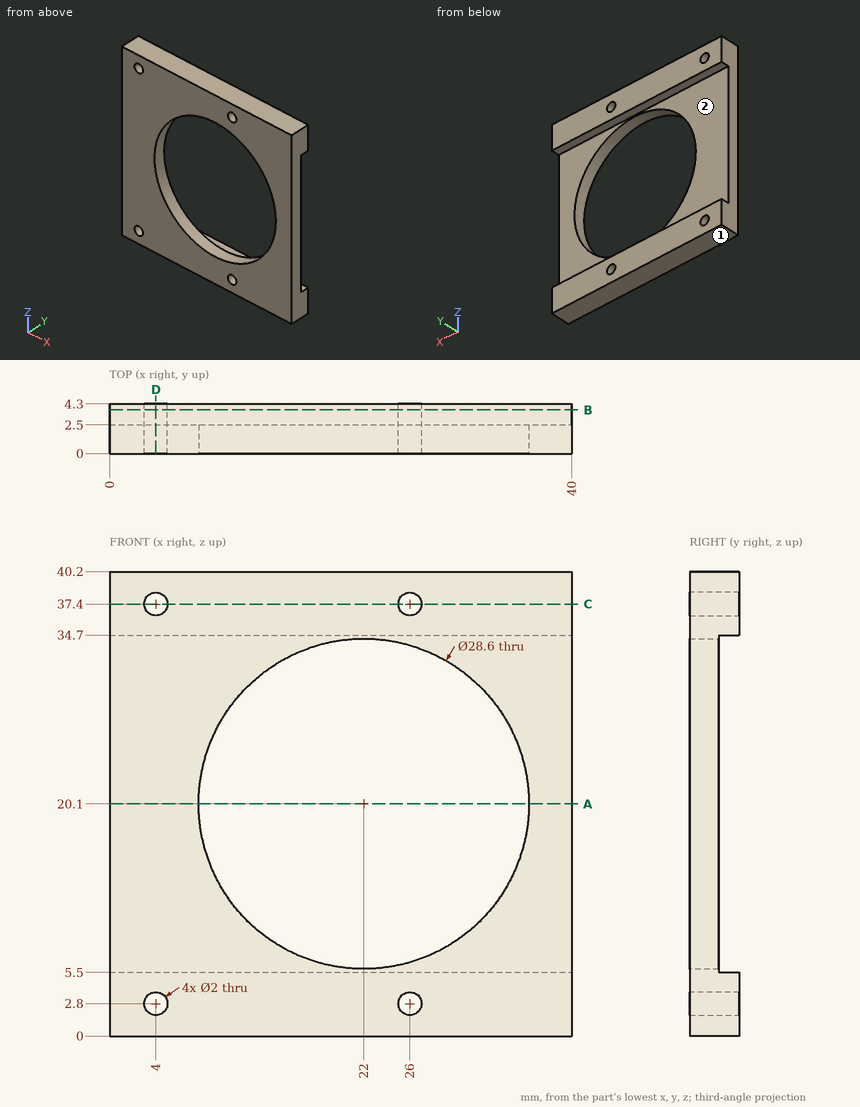
Design review of the part shown in the three views and the two pictorial views. Dimensions are in mm from the part's minimum x, y and z. A direction names the side the tool comes from. Coordinates: 2 decimals unless noted, no trailing zeros. Write each loop counter-clockwise with the first axis right and the second up, starting at its lowest first coordinate (ties: lowest second). Pieces come first, ordered by that corner, then holes.
(1) Add section B-B on y = 3.8. Give the boundary of the cut face in (x, z), then the cut area to 3 significant figures.
(2) For pin 1 Ø1 at (x, z) = (18.5, 32.5) entering from -Y, flat-tipped, find the tip position at first contact; note if it passes through.
(3) Add section C-C on z = 37.4. Give the boundary of the cut face in (x, y), then the cut area to 3 significant figures.
(4) Add section A-A on z = 20.1. Give the boundary of the cut face in (x, y), then the cut area to 3 significant figures.
(5) Add section D-D on x = 4. Give the boundary of the cut face in (y, z).
(6) Wall thickness on probe 1 along X at (y, z) = (2.95, 2.8); probe 2 along X at (y, z) = (1.65, 20.1); probe 3 along Z at (x, y) = (7.5, 3.1): over which ranges is each line inside the solid? List them lowest first.
(7) Tool access review of the marked faces 1 and 2: name each direction out of +Z, -Z, +X, -X, +Y, -Y from which nothing blocks a thin tool from reaching the whole face with its end or side.
Answer sheet:
1. outline: (0, 0) - (40, 0) - (40, 5.5) - (0, 5.5) - close; (0, 34.7) - (40, 34.7) - (40, 40.2) - (0, 40.2) - close; hole circle Ø2 at (4, 2.8); hole circle Ø2 at (4, 37.4); hole circle Ø2 at (26, 2.8); hole circle Ø2 at (26, 37.4)
1. area: 427 mm2
2. pin 1: passes through
3. outline: (0, 0) - (3, 0) - (3, 4.3) - (0, 4.3) - close; (5, 0) - (25, 0) - (25, 4.3) - (5, 4.3) - close; (27, 0) - (40, 0) - (40, 4.3) - (27, 4.3) - close
3. area: 155 mm2
4. outline: (0, 0) - (7.7, 0) - (7.7, 2.5) - (0, 2.5) - close; (36.3, 0) - (40, 0) - (40, 2.5) - (36.3, 2.5) - close
4. area: 28.5 mm2
5. outline: (0, 0) - (4.3, 0) - (4.3, 1.8) - (0, 1.8) - close; (0, 3.8) - (4.3, 3.8) - (4.3, 5.5) - (2.5, 5.5) - (2.5, 34.7) - (4.3, 34.7) - (4.3, 36.4) - (0, 36.4) - close; (0, 38.4) - (4.3, 38.4) - (4.3, 40.2) - (0, 40.2) - close
6. probe 1: x = 0 to 3, 5 to 25, 27 to 40
6. probe 2: x = 0 to 7.7, 36.3 to 40
6. probe 3: z = 0 to 5.5, 34.7 to 40.2
7. face 1: -Z, +X, -X, +Y, -Y
7. face 2: +X, -X, +Y
